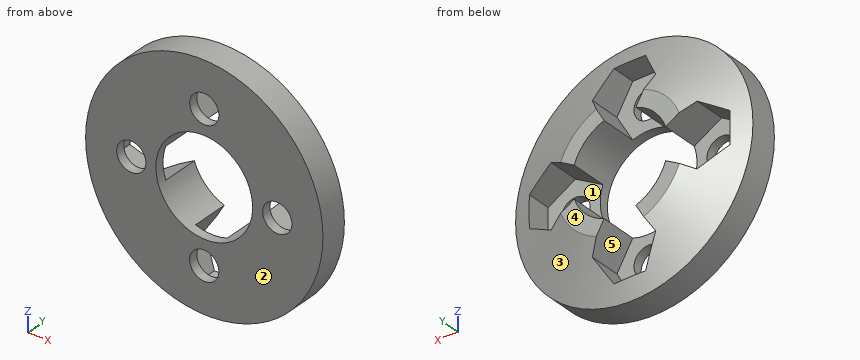
from build123d import *

# Parameters (mm, degrees)
CUT_EXTRUDE_1_DEPTH      = 4.5
CUT_EXTRUDE_1_DEPTH_BACK = 3.5
SKETCH_6_R               = 1.6
CUT_EXTRUDE_2_DEPTH      = 20.189841062
CUT_EXTRUDE_START        = 10
SKETCH_8_R               = 5.3
CUT_EXTRUDE_3_DEPTH      = 10


with BuildPart() as part:
    # 草图2 → 旋转1 (revolve)
    with BuildSketch(Plane.XY, mode=Mode.PRIVATE) as revolve_1_sk:
        Polygon((0, 0), (-13, 0), (-13, 3), (-7, 5), (-5.3, 5), (-5.3, 3), (0, 3), (0, 1.5), align=None)
    revolve(revolve_1_sk.sketch.rotate(Axis((0, 0, 0), (0, 1, 0)), 180), axis=Axis((0, 0, 0), (0, 1, 0)))

    # 草图5 → 切除-拉伸1 (cut, two sides: drawn at the far end of the back side and taken through both)
    with BuildSketch(Plane(origin=(0, 5.5, 0), x_dir=(-1, 0, 0), z_dir=(0, -1, 0)).offset(-CUT_EXTRUDE_1_DEPTH_BACK)):
        Polygon((8, -3.464101615), (11, -1.732050808), (11, 1.732050808), (8, 3.464101615), (5, 1.732050808), (5, -1.732050808), align=None)
        Polygon((3.464101615, 8), (1.732050808, 11), (-1.732050808, 11), (-3.464101615, 8), (-1.732050808, 5), (1.732050808, 5), align=None)
        Polygon((-3.464101615, -8), (-1.732050808, -11), (1.732050808, -11), (3.464101615, -8), (1.732050808, -5), (-1.732050808, -5), align=None)
        Polygon((-8, 3.464101615), (-11, 1.732050808), (-11, -1.732050808), (-8, -3.464101615), (-5, -1.732050808), (-5, 1.732050808), align=None)
    extrude(amount=CUT_EXTRUDE_1_DEPTH + CUT_EXTRUDE_1_DEPTH_BACK, mode=Mode.SUBTRACT)

    # 草图6 → 切除-拉伸2 (cut, through all)
    with BuildSketch(Plane(origin=(0, 5.5, 0), x_dir=(-1, 0, 0), z_dir=(0, -1, 0))):
        with Locations((0, 8)):
            Circle(SKETCH_6_R)
        with Locations((8, 0)):
            Circle(SKETCH_6_R)
        with Locations((0, -8)):
            Circle(SKETCH_6_R)
        with Locations((-8, 0)):
            Circle(SKETCH_6_R)
    extrude(amount=CUT_EXTRUDE_2_DEPTH, mode=Mode.SUBTRACT)

    # 草图8 → 切除-拉伸3 (cut)
    with BuildSketch(Plane(origin=(0, 5.5, 0), x_dir=(-1, 0, 0), z_dir=(0, -1, 0)).offset(CUT_EXTRUDE_START)):
        with Locations(Location((0, 0, 0), (0, 0, 160.875716495))):
            Circle(SKETCH_8_R)
    extrude(amount=-CUT_EXTRUDE_3_DEPTH, mode=Mode.SUBTRACT)


solid = part.part
The listing builds one solid part. Answer for the finished solid, in the listing's coordinates (mm). Face numbers are marked on the shaded views. A direction names the side the tool comes from. Give positions to 0.01 mm unless a question says otherwise; leave off trailing zeros. Write each loop counter-clockwise with the first axis right and the second up, starting at its lowest first coordinate (ties: lowest second). Pieces come first, ordered by that corner, then holes.
1) Given P1, Ø1.5, axis at x = 9, z = -5.5, coming from the +Y side; P2, Ø0.8, axis at x = -1, y = 3, coming from the -Z side; P3, Ø5, axis at x = -8, z = 0, coming from the +Y side, each flat-ended and moving along its own axis, determine where each tip first touches the part or whether it passes through.
2) Find the intervals of material crossed by L1, parallel to Z at x = 0, y = 0.75; L2, parallel to X at y = 2.65, z = 0.25; L3, parallel to X at y = 1.9, z = -1.5, in increasing order.
3) Section B-B (z = 0) is taken. Write down the section's boundary in (x, y).
4) A tool of negligible diameter and unlimited length cuts with its end or side. For the marked faces 1 and 2, from which of +Z, -Z, +X, -X, +Y, -Y can it reach the whole face along a straight path? Write none if from no direction.
5) For a pull along Z with two mould halves and no side action, classify the marked faces 3, 4 and 5 as pulls with the +Z half, pulls with the -Z half, needs draft (parallel to the pull), parting line crosses it, or undercut.
6) Section A-A (x = 0) is taken. Write down the section's boundary in (y, z).
Response:
1. P1: stops at y = 4.07
1. P2: stops at z = -12.99
1. P3: stops at y = 1
2. L1: z = -13 to -9.6, -6.4 to -5.3, 5.3 to 6.4, 9.6 to 13
2. L2: x = -13 to -11, 11 to 13
2. L3: x = -12.91 to -11, 11 to 12.91
3. outline: (-13, 0) - (-9.6, 0) - (-9.6, 1) - (-11, 1) - (-11, 3.67) - (-13, 3) - close; (-6.4, 0) - (-5.3, 0) - (-5.3, 1) - (-6.4, 1) - close; (5.3, 0) - (6.4, 0) - (6.4, 1) - (5.3, 1) - close; (9.6, 0) - (13, 0) - (13, 3) - (11, 3.67) - (11, 1) - (9.6, 1) - close
4. face 1: +Y
4. face 2: +Z, -Z, +X, -X, -Y
5. face 3: parting line crosses it
5. face 4: needs draft
5. face 5: undercut
6. outline: (0, -13) - (3, -13) - (3.67, -11) - (1, -11) - (1, -9.6) - (0, -9.6) - close; (0, -6.4) - (1, -6.4) - (1, -5.3) - (0, -5.3) - close; (0, 5.3) - (1, 5.3) - (1, 6.4) - (0, 6.4) - close; (0, 9.6) - (1, 9.6) - (1, 11) - (3.67, 11) - (3, 13) - (0, 13) - close
